Check sheet for the drawn part. Datum: minimum x, y, z corner. Units: mm. A direction names the side the tool comes from. Round coordinates to 2 decimals unless told otherwise and drop trailing zeros. Write each loop counter-clockwise with the first axis right and the second up, starting at its lowest first coordinate (ties: lowest second). Pieces come first, ordered by that corner, then holes. Notation, with made-up numbers: (-16.75, 54) - (-5.75, 54) arc R10 cw to (-5.75, 70) - close; hole circle Ø1 at (77.5, -26). An arc over 180 degrees is marked (long way). Answer as a JSON object with one key per item and string values. Group by question number.
1) Section check C-C (y = 27.5). Enter the section's corners in (x, z), then the cut area to 3 significant figures.
2) Go/stop test with flat-tipped pins: pin 1 Ø13 at (x, z) = (4.5, 39) entering from -Y; pin 2 Ø12 at (y, z) = (28.5, 23) entering from +X; pin 3 Ø11.5 at (x, z) = (23, 22.5) entering from -Y; pin 4 Ø8 at (y, z) = (49.5, 25) entering from -X. Record where each tip stops, or that it passes through.
3) Thickness scan on line 1 (X direction, y = 0.55, z = 11.5); line 2 (Z direction, x = 27.5, y = 1.15). Record the ranges inside material, lowest first.
4) Set-up check for the marked faces 1, 2 and 3: record each of +Z, -Z, +X, -X, +Y, -Y from which the full face is reachable in a straight line by a thin tool's end or side.
5) Section check B-B (z = 46.5). Enter the section's corners in (x, y).
6) Section check D-D (z = 32). Enter the section's corners in (x, y), then the cut area to 3 significant figures.
7) Mould release check, pull along X, two halves, no side actions. Record for the marked faces 4, 5 and 6: +X half, -X half, draft (parallel to the pull), parting line (faces both ways), or undercut.
8) Section check A-A (x = 27.5). Enter the section's corners in (y, z), then the cut area to 3 significant figures.
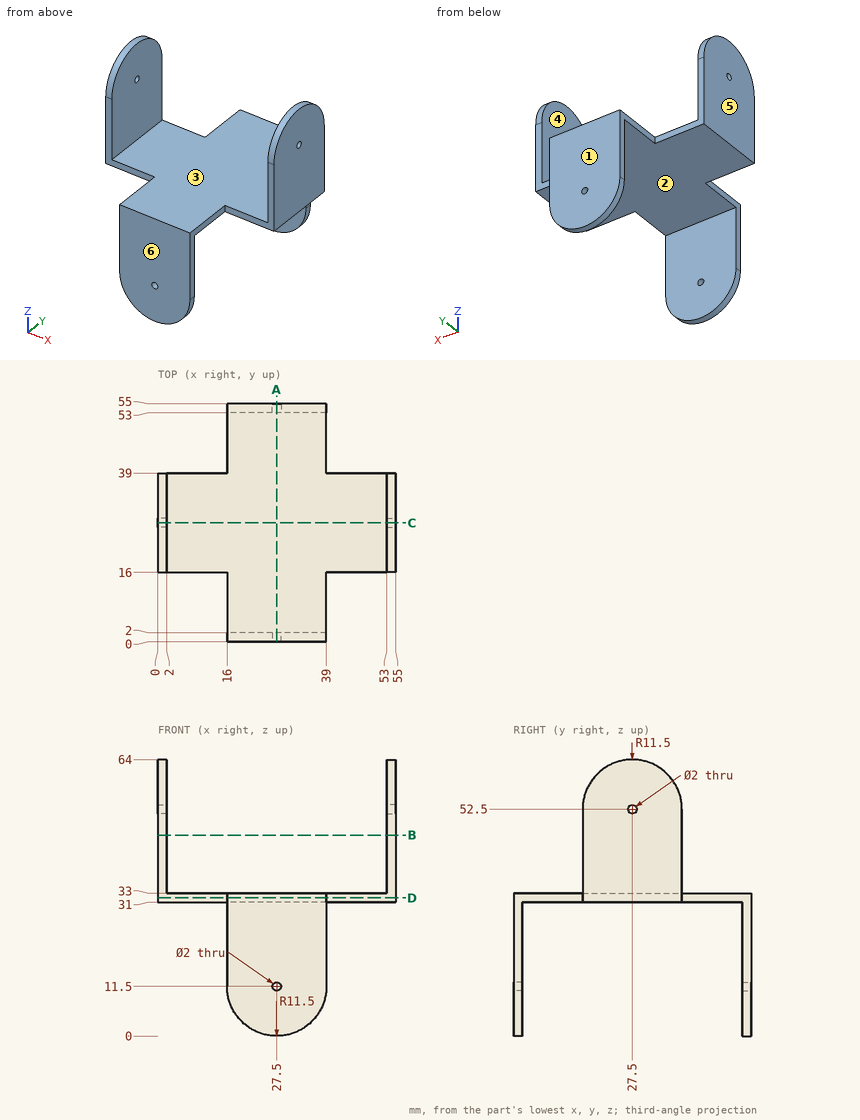
Returned:
{
 "1": {"outline": "(0, 31) - (55, 31) - (55, 51.5) - (53, 51.5) - (53, 33) - (2, 33) - (2, 51.5) - (0, 51.5) - close; (0, 53.5) - (2, 53.5) - (2, 64) - (0, 64) - close; (53, 53.5) - (55, 53.5) - (55, 64) - (53, 64) - close", "area": "226 mm2"},
 "2": {"pin 1": "y = 16", "pin 2": "through", "pin 3": "y = 0", "pin 4": "x = 16"},
 "3": {"line 1": "16 to 26.5, 28.5 to 39", "line 2": "0 to 10.5, 12.5 to 33"},
 "4": {"face 1": "+Z, -Z, +X, -X, +Y", "face 2": "-Z, +X, -X", "face 3": "+Z, +Y, -Y"},
 "5": {"outline": "(0, 16) - (2, 16) - (2, 39) - (0, 39) - close; (53, 16) - (55, 16) - (55, 39) - (53, 39) - close"},
 "6": {"outline": "(0, 16) - (16, 16) - (16, 0) - (39, 0) - (39, 16) - (55, 16) - (55, 39) - (39, 39) - (39, 55) - (16, 55) - (16, 39) - (0, 39) - close", "area": "2,000 mm2"},
 "7": {"face 4": "undercut", "face 5": "-X half", "face 6": "draft"},
 "8": {"outline": "(0, 0) - (2, 0) - (2, 10.5) - (0, 10.5) - close; (0, 12.5) - (2, 12.5) - (2, 31) - (53, 31) - (53, 12.5) - (55, 12.5) - (55, 33) - (0, 33) - close; (53, 0) - (55, 0) - (55, 10.5) - (53, 10.5) - close", "area": "226 mm2"}
}
